Input: dimensioned drawing with shaded views. Units: mm. Origin: part minimum x, y, z. A direction names the side the tool comes from. Give positions to 0.01 mm unless a question says otherwise; leave off trailing zeros. Loops run counter-clockwise (first coordinate to the right, second up) from the corner with the lowest first, then second, coordinate; pieces in that order, holes last. Notation, with made-up numbers: (77, 36.25) -> (115, 36.25) arc R13 ccw to (115, 59.25) -> close; hole circle Ø5 at (60, 44.5). An arc over 180 degrees is marked (long way). Answer in a Markdown table with one row per item. Add a question column.
1) Line query: line 1 (Y direction, x = 0.35, z = 4.75) (1 decimal); line 2 (Z direction, x = 3.25, y = 5.75); line 3 (Y direction, x = 3.8, z = 4) (1 decimal). Output: solid intervals per line, ascending. Write a range as from..to.
2) Section query B-B (x = 1). Return the cut outline in (y, z), plus the area to 3 significant figures.
3) Section query A-A (x = 0.5). Return the cut outline in (y, z) (1 decimal).
4) Draft query along Y for the marked faces 1, 2 and 3. Return one class per face: +Y half, -Y half, draft (parallel to the pull), parting line (faces both ways), or undercut.
5) Access query for the marked faces 4 and 5. Directions: +Z, -Z, +X, -X, +Y, -Y. A direction counts if a zero-diameter tool reaches every point of the face in a straight line with its end or side. Return the directions, or none.
6) Section query C-C (x = 4.2). Return the cut outline in (y, z).
7) First-contact query: P1, Ø1.5, axis at x = 4, z = 4, coming from the +Y side; P2, Ø1, axis at x = 4, y = 5, coming from the +Z side. Flat tips, straight axial feed; report the tip coordinate or a pass-through.
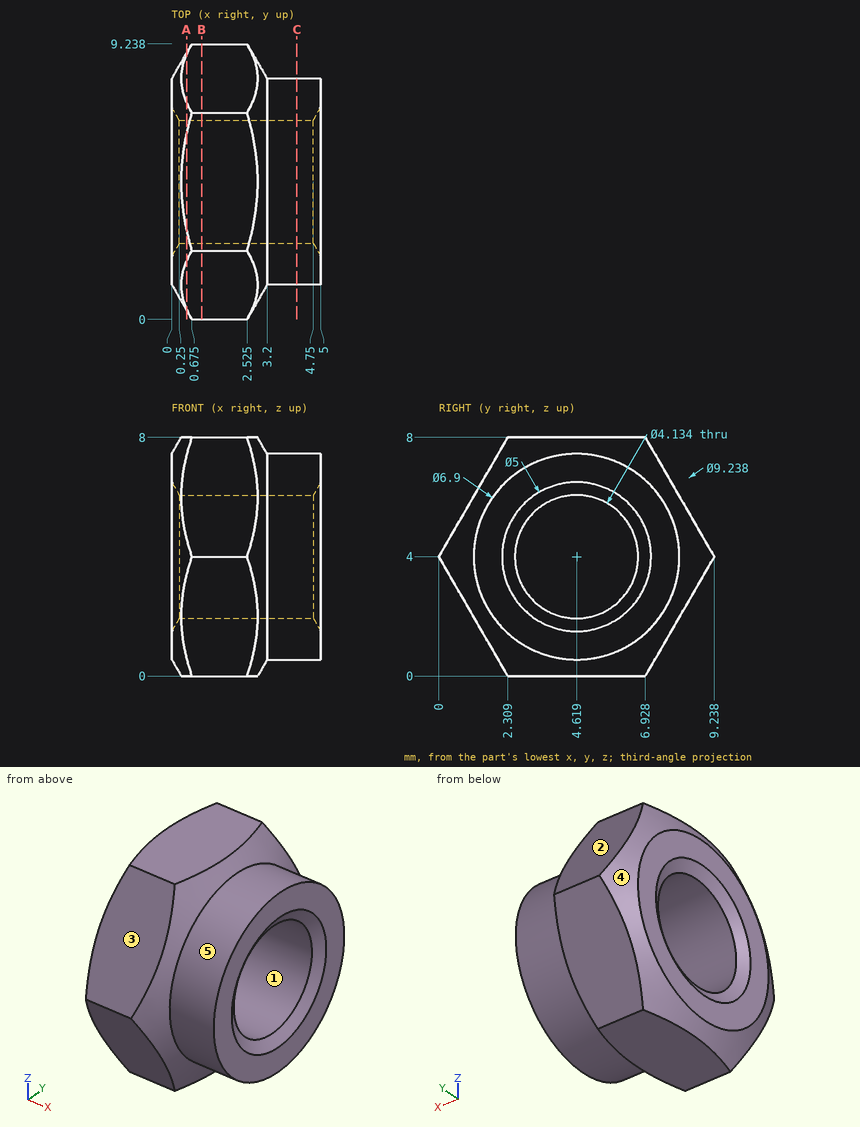
Evaluation:
| question | item | result |
|---|---|---|
| 1 | line 1 | 0.6..2.7, 6.5..8.6 |
| 1 | line 2 | 0.74..2.27, 5.73..7.26 |
| 1 | line 3 | 1.2..2.6, 6.7..8.1 |
| 2 | outline | (0, 4) -> (2.31, 0) -> (6.93, 0) -> (9.24, 4) -> (6.93, 8) -> (2.31, 8) -> close; hole circle Ø4.13 at (4.62, 4) |
| 2 | area | 42.0 mm² |
| 3 | outline | (0.3, 3.4) -> (2, 0.6) arc R4.3 ccw to (3, 0) -> (6.2, 0) arc R4.3 ccw to (7.3, 0.6) -> (8.9, 3.4) arc R4.3 ccw to (8.9, 4.6) -> (7.3, 7.4) arc R4.3 ccw to (6.2, 8) -> (3, 8) arc R4.3 ccw to (2, 7.4) -> (0.3, 4.6) arc R4.3 ccw to start; hole circle Ø4.1 at (4.6, 4) |
| 4 | face 1 | undercut |
| 4 | face 2 | +Y half |
| 4 | face 3 | -Y half |
| 5 | face 4 | -X |
| 5 | face 5 | +X |
| 6 | outline | circle Ø6.9 at (4.62, 4); hole circle Ø4.13 at (4.62, 4) |
| 7 | P1 | y = 8.07 |
| 7 | P2 | z = 7.45 |
